Part print with two shaded views. Sizes in mm from the minimum x, y, z corner. Coordinates: 2 decimals unless noted, no trailing zeros. Loops run counter-clockwise (first coordinate to the right, second up) from the corner with the lowest first, then second, coordinate; pieces in that order, holes last. Notation, with made-up numbers: (-23.75, 25.5) -> (32.25, 25.5) arc R25 cw to (32.25, 57.5) -> close; hole circle Ø1 at (16, 57.25). An arc over 180 degrees is marked (long way). One line per item, written item: value. Start each with the question number.
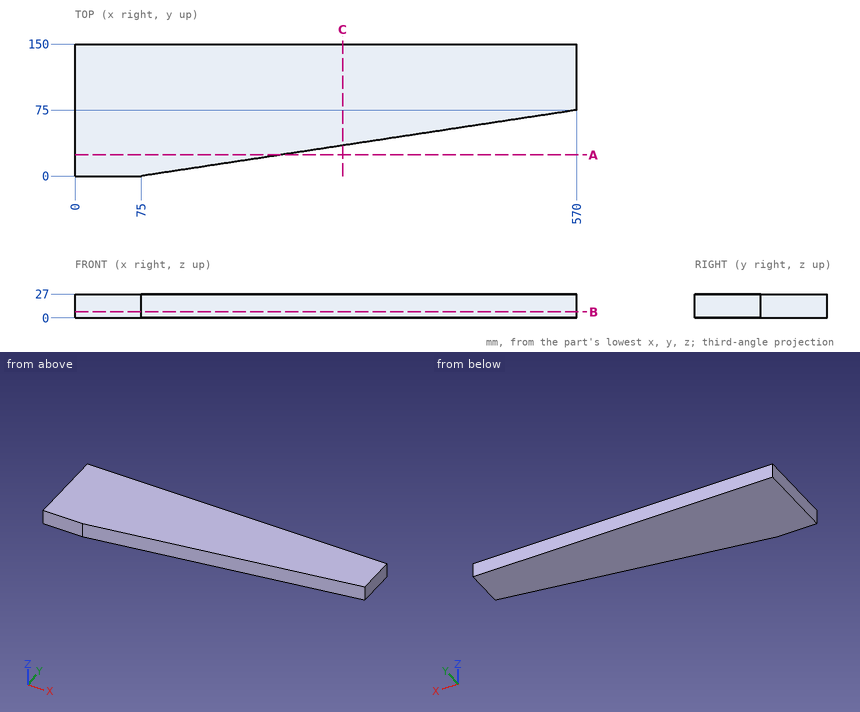
Item 1: Probe probe 1 along Y at (x, z) = (218.5, 22.5); probe 2 along Y at (x, z) = (165, 17.5). List the from-to ranges inside material, lowest first.
Item 2: Band-saw the part on C-C, the plane x = 304. List the corners of the cut face in (y, z), and give its area (3 significant figures).
Item 3: Band-saw the part on B-B, the plane z = 6.75. List the corners of the cut face in (x, y), and give its area (3 significant figures).
Item 4: Band-saw the part on A-A, the plane y = 24. List the corners of the cut face in (x, z).
Item 5: Drop flat-ended pins along their axis: pin 1 Ø5 at (x, z) = (484.5, 19) entering from -Y; pin 2 Ø10 at (x, z) = (244, 12.5) entering from -Y. Give the stop position or say it passes through.
Worked out:
1. probe 1: y = 21.74 to 150
1. probe 2: y = 13.64 to 150
2. outline: (34.7, 0) -> (150, 0) -> (150, 27) -> (34.7, 27) -> close
2. area: 3,110 mm²
3. outline: (0, 0) -> (75, 0) -> (570, 75) -> (570, 150) -> (0, 150) -> close
3. area: 66,900 mm²
4. outline: (0, 0) -> (233.4, 0) -> (233.4, 27) -> (0, 27) -> close
5. pin 1: stops at y = 61.67
5. pin 2: stops at y = 24.85
